```python
from build123d import *

# Parameters (mm, degrees)
F1_DEPTH = 25.4


with BuildPart() as f1:
    # F0 (on Top) → F1 (new body)
    with BuildSketch(Plane.XY):
        Polygon((38.1, 76.2), (22.8934809566, 45.7869619131), (53.3065190434, 45.7869619131), align=None)
        Polygon((22.8934809566, 45.7869619131), (0, 45.7869619131), (17.6044199078, 35.2088398157), align=None)
        Polygon((17.6044199078, 35.2088398157), (0, 0), (38.1, 22.8934809566), align=None)
        Polygon((38.1, 22.8934809566), (76.2, 0), (58.5955800922, 35.2088398157), align=None)
        Polygon((58.5955800922, 35.2088398157), (76.2, 45.7869619131), (53.3065190434, 45.7869619131), align=None)
        Polygon((17.6044199078, 35.2088398157), (38.1, 22.8934809566), (58.5955800922, 35.2088398157), (53.3065190434, 45.7869619131), (22.8934809566, 45.7869619131), align=None)
    extrude(amount=F1_DEPTH)


solid = f1.part
```
For this review, take the finished solid that the model builds, in its own axes (mm). A direction names the side the tool comes from. Round coordinates to 2 decimals unless told otherwise and drop trailing zeros. Order: outer loops, then holes, each group sorted by start corner. A loop starts at its lowest first (then second) coordinate and runs counter-clockwise, first axis right, second up.
Q1. Insertion check: P1, Ø1.5, axis at x = 47, z = 6.5, coming from the +Y side; P2, Ø5, axis at x = 34, z = 11, coming from the +Y side; P3, Ø8, axis at y = 36, z = 22, coming from the +X side. Each pin has a flat end and moves straight along its axis. Give the tip position at first contact, or say it passes through.
Findings below:
P1: stops at y = 59.9
P2: stops at y = 73
P3: stops at x = 66.57
Q2. We need section B-B, the plane z = 23. Give the boundary of the cut face in (x, y).
Findings below:
outline: (0, 0) - (38.1, 22.89) - (76.2, 0) - (58.6, 35.21) - (76.2, 45.79) - (53.31, 45.79) - (38.1, 76.2) - (22.89, 45.79) - (0, 45.79) - (17.6, 35.21) - close
Q3. We need section A-A, the plane x = 62.5. Give the boundary of the cut face in (y, z).
Findings below:
outline: (8.23, 0) - (27.4, 0) - (27.4, 25.4) - (8.23, 25.4) - close; (37.55, 0) - (45.79, 0) - (45.79, 25.4) - (37.55, 25.4) - close
Q4. We need section C-C, the plane y = 9.5. Give the boundary of the cut face in (x, z), plus the area to 3 significant figures.
Findings below:
outline: (4.75, 0) - (15.81, 0) - (15.81, 25.4) - (4.75, 25.4) - close; (60.39, 0) - (71.45, 0) - (71.45, 25.4) - (60.39, 25.4) - close
area: 562 mm2
Q5. Machinability: for faces 1 (the flat face through (8.68, 40.57, 12.52)), 2 (the flat face through (18.783, 11.286, 12.522)), 3 (the flat face through (12, 45.787, 13)), 4 (the flat face through (65, 45.787, 13)), 5 (the flat face through (67.5, 17.4, 12.5)), which of the approach directions +Z, -Z, +X, -X, +Y, -Y give a long, thin tool a straight path to every point of the face, cutting with its end or side? Answer none if there is none.
Findings below:
face 1: +Z, -Z, -X
face 2: +Z, -Z, -Y
face 3: +Z, -Z, -X, +Y
face 4: +Z, -Z, +X, +Y
face 5: +Z, -Z, +X
Q6. Wall thickness on line 1 (Y direction, x = 7.5, z = 13); line 2 (Y direction, x = 65.5, z = 13.25); line 3 (X direction, y = 4.5, z = 21): over which ranges is each line inside the solid? List them lowest first.
Findings below:
line 1: y = 4.51 to 15, 41.28 to 45.79
line 2: y = 6.43 to 21.4, 39.36 to 45.79
line 3: x = 2.25 to 7.49, 68.71 to 73.95
Q7. Mouldability with a two-part tool opening along Y and no side actions: class faces 6 (the flat face through (45.8, 60.8, 12.5)), 7 (the flat face through (56.88, 11.61, 12.52)), 8 (the flat face through (67.27, 40.42, 12.52)) as pulls with the +Y half, pulls with the -Y half, needs draft (parallel to the pull), parting line crosses it, or undercut.
Findings below:
face 6: pulls with the +Y half
face 7: pulls with the -Y half
face 8: undercut
Q8. We need section D-D, the plane y = 59.5. Give the boundary of the cut face in (x, z).
Findings below:
outline: (29.75, 0) - (46.45, 0) - (46.45, 25.4) - (29.75, 25.4) - close
